from build123d import *

# Parameters (mm, degrees)
F1_DEPTH       = 30
F2_R           = 10
F3_D           = 12.6
F3_CBORE_D     = 19.25
F3_CBORE_DEPTH = 12


with BuildPart() as f1:
    # F0 (on Front) → F1 (new body)
    with BuildSketch(Plane.XZ):
        Polygon((0, -40), (0, 0), (30, 30), (60, 30), (60, 60), (-50, 60), (-50, -40), align=None)
    extrude(amount=-F1_DEPTH)

    # F2
    f2_edges = [f1.edges().sort_by_distance(p)[0] for p in [
        (-50, 15, -40),
        (0, 15, -40),
        (-50, 15, 60),
        (60, 15, 60),
        (60, 15, 30),
    ]]
    fillet(f2_edges, radius=F2_R)

    # F3 (through all)
    with Locations(Plane.XZ):
        with Locations((45, 45)):
            CounterBoreHole(F3_D / 2, F3_CBORE_D / 2, F3_CBORE_DEPTH)


solid = f1.part
Source: CAD feature listing. Evaluate the final solid. Frame: model axes, mm. A direction names the side the tool comes from. Give positions to 0.01 mm unless a question says otherwise; leave off trailing zeros. Write each loop counter-clockwise with the first axis right and the second up, starting at its lowest first coordinate (ties: lowest second). Pieces come first, ordered by that corner, then holes. Notation, with made-up numbers: M 75.5,58.25 L 87.5,58.25 A20 cw 87.5,73.25 Z; hole C 11.5,65.25 d10. An arc over 180 degrees is marked long. Answer as a JSON object with one key per item and string values.
Q1. Cut plane D-D, the plane y = 18.25. Return the cut outline in (x, z), then the cut area to 3 significant figures.
Geometry check:
{"outline": "M -50,-30 A10 ccw -40,-40 L -10,-40 A10 ccw 0,-30 L 0,0 L 30,30 L 50,30 A10 ccw 60,40 L 60,50 A10 ccw 50,60 L -40,60 A10 ccw -50,50 Z; hole C 45,45 d12.6", "area": "7,020 mm^2"}
Q2. Contact query for flat-ended pins moving along their axis: P1, Ø16, axis at x = 40, y = 18, coming from the -Z side; P2, Ø9.5, axis at x = 45, z = 49, coming from the -Y side; P3, Ø5, axis at y = 17.5, z = 34.5, coming from the +X side; P4, Ø10, axis at x = -17, z = 40.5, coming from the -Y side. Output: stop coordinate, or through.
Geometry check:
{"P1": "stops at z = 30", "P2": "stops at y = 12", "P3": "stops at x = 59.54", "P4": "stops at y = 0"}
Q3. Ray query, line 1 along Z through (x, y) = (45, 2.5) (3 decimals); line 2 along Z through (x, y) = (45, 25.75); line 3 along X through (y, z) = (20.25, 46). Return the intervals inside material, ascending.
Geometry check:
{"line 1": "z = 30 to 35.375, 54.625 to 60", "line 2": "z = 30 to 38.7, 51.3 to 60", "line 3": "x = -50 to 38.78, 51.22 to 60"}
Q4. Cut plane C-C, the plane x = 45. Return the cut outline in (y, z) (3 decimals), then the cut area to 3 significant figures.
Geometry check:
{"outline": "M 0,30 L 30,30 L 30,38.7 L 12,38.7 L 12,35.375 L 0,35.375 Z; M 0,54.625 L 12,54.625 L 12,51.3 L 30,51.3 L 30,60 L 0,60 Z", "area": "442 mm^2"}
Q5. Mould query, pull axis X, two halves, no side actions, for faces 1 (the face through (56.99, 15.21, 32.85)), 2 (the face through (47, 12, 38.7)), 3 (the face through (-8, 30, 22)). Classes: +X half, -X half, draft (parallel to the pull), parting line (faces both ways), or undercut.
Geometry check:
{"face 1": "+X half", "face 2": "undercut", "face 3": "draft"}
Q6. Cut plane B-B, the plane y = 3.25. Return the cut outline in (x, z) (3 decimals), then the cut area to 3 significant figures.
Geometry check:
{"outline": "M -50,-30 A10 ccw -40,-40 L -10,-40 A10 ccw 0,-30 L 0,0 L 30,30 L 50,30 A10 ccw 60,40 L 60,50 A10 ccw 50,60 L -40,60 A10 ccw -50,50 Z; hole C 45,45 d19.25", "area": "6,850 mm^2"}
Q7. Access query for faces 4 (the face through (49.64, 21.13, 49.26)), 5 (the face through (0, 15, -15)), 6 (the face through (49.44, 5.92, 36.46)). Directions: +Z, -Z, +X, -X, +Y, -Y. A direction counts if a zero-diameter tool reaches every point of the face in a straight line with its end or side. Return the directions, or none.
Geometry check:
{"face 4": "+Y, -Y", "face 5": "-Z, +X, +Y, -Y", "face 6": "-Y"}
Q8. Cut plane A-A, the plane z = 45. Return the cut outline in (x, y) (3 decimals), then the cut area to 3 significant figures.
Geometry check:
{"outline": "M -50,0 L 35.375,0 L 35.375,12 L 38.7,12 L 38.7,30 L -50,30 Z; M 51.3,12 L 54.625,12 L 54.625,0 L 60,0 L 60,30 L 51.3,30 Z", "area": "2,840 mm^2"}
